from build123d import *

# Parameters (mm, degrees)
SKETCH1_W           = 25.4
SKETCH1_H           = 50.8
SKETCH1_W_2         = 19.05
SKETCH1_H_2         = 44.45
BOSS_EXTRUDE1_DEPTH = 279.4
CUT_EXTRUDE1_DEPTH  = 279.4


with BuildPart() as part:
    # Sketch1 → Boss-Extrude1 (new body)
    with BuildSketch(Plane(origin=(0, 0, 0), x_dir=(1, 0, 0), z_dir=(0, 1, 0))):
        with Locations((12.7, 25.4)):
            Rectangle(SKETCH1_W, SKETCH1_H)
        with Locations((12.7, 25.4)):
            Rectangle(SKETCH1_W_2, SKETCH1_H_2, mode=Mode.SUBTRACT)
    extrude(amount=BOSS_EXTRUDE1_DEPTH)

    # Sketch2 → Cut-Extrude1 (cut)
    with BuildSketch(Plane(origin=(25.4, 0, 0), x_dir=(0, 0, -1), z_dir=(1, 0, 0))):
        Polygon((0, 279.4), (50.8, 228.6), (50.8, 279.4), align=None)
    extrude(amount=-CUT_EXTRUDE1_DEPTH, mode=Mode.SUBTRACT)


solid = part.part
Input: part model. Units: mm. Frame: model coordinates. A direction names the side the tool comes from. Round coordinates to 2 decimals unless told otherwise and drop trailing zeros. Order: outer loops, then holes, each group sorted by start corner. A loop starts at its lowest first (then second) coordinate and runs counter-clockwise, first axis right, second up.
1. Cut plane D-D, the plane y = 260. Output: boundary loops of the cut face in (x, z) (3 decimals).
The answers:
outline: (0, -19.4) - (3.175, -19.4) - (3.175, -3.175) - (22.225, -3.175) - (22.225, -19.4) - (25.4, -19.4) - (25.4, 0) - (0, 0) - close
2. Cut plane B-B, the plane x = 17.75. Output: boundary loops of the cut face in (y, z) (3 decimals), then the cut area to 3 significant figures.
The answers:
outline: (0, -50.8) - (228.6, -50.8) - (231.775, -47.625) - (0, -47.625) - close; (0, -3.175) - (276.225, -3.175) - (279.4, 0) - (0, 0) - close
area: 1,610 mm2
3. Cut plane C-C, the plane y = 113.5. Output: boundary loops of the cut face in (x, z) (3 decimals), then the cut area to 3 significant figures.
The answers:
outline: (0, -50.8) - (25.4, -50.8) - (25.4, 0) - (0, 0) - close; hole (3.175, -47.625) - (22.225, -47.625) - (22.225, -3.175) - (3.175, -3.175) - close
area: 444 mm2
4. Mould query, pull axis X, two halves, no side actions, for faces 1 (the face through (0, 138, -25)), 2 (the face through (13, 113, -50.8)), 3 (the face through (13, 114, -47.625)). Classes: released by +X, released by -X, zero draft, split by the parting line, or undercut.
The answers:
face 1: released by -X
face 2: zero draft
face 3: undercut
5. Pin query (flat end, axial travel): P1, Ø8, axis at x = 3.5, z = -33.5, coming from the +Y side. Return the tip coordinate at first contact, or that it passes through.
The answers:
P1: stops at y = 249.89
6. Material intervals for line 1 (Z direction, x = 7.75, y = 110.5) (3 decimals); line 2 (X direction, y = 117, z = -17) (3 decimals); line 3 (Z direction, x = 6.5, y = 254) (3 decimals), sorted ascending.
The answers:
line 1: z = -50.8 to -47.625, -3.175 to 0
line 2: x = 0 to 3.175, 22.225 to 25.4
line 3: z = -3.175 to 0
7. Cut plane A-A, the plane z = -10. Output: boundary loops of the cut face in (x, y) (3 decimals), then the cut area to 3 significant figures.
The answers:
outline: (0, 0) - (3.175, 0) - (3.175, 269.4) - (0, 269.4) - close; (22.225, 0) - (25.4, 0) - (25.4, 269.4) - (22.225, 269.4) - close
area: 1,710 mm2
8. Set-up query: faces 4 (the face through (2, 0, -24)), 5 (the face through (22.225, 136, -25)). Return all of +Z, -Z, +X, -X, +Y, -Y with unobstructed straight access to the full face (end or side cutting, diameter ignored); none if empty.
The answers:
face 4: +Z, -Z, +X, -X, -Y
face 5: +Y, -Y
